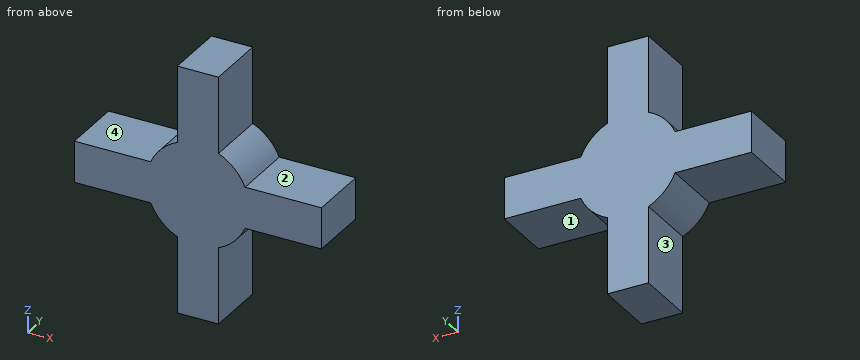
```python
from build123d import *

# Parameters (mm, degrees)
F0_W     = 76.2
F0_H     = 76.2
F2_DEPTH = 19.05
F1_W     = 31.75
F1_H     = 31.75
F3_DEPTH = 19.051
F4_R     = 15.875
F5_DEPTH = 19.05


with BuildPart() as f2:
    # F0 (on Front) → F2 (new body)
    with BuildSketch(Plane.XZ):
        Rectangle(F0_W, F0_H)
    extrude(amount=F2_DEPTH)

    # F1 (on Front) → F3 (cut, through all)
    with BuildSketch(Plane.XZ):
        with Locations((-22.225, 22.225)):
            Rectangle(F1_W, F1_H)
        with Locations((-22.225, -22.225)):
            Rectangle(F1_W, F1_H)
        with Locations((22.225, -22.225)):
            Rectangle(F1_W, F1_H)
        with Locations((22.225, 22.225)):
            Rectangle(F1_W, F1_H)
    extrude(amount=F3_DEPTH, mode=Mode.SUBTRACT)

    # F4 (on Front) → F5 (join)
    with BuildSketch(Plane.XZ):
        Circle(F4_R)
    extrude(amount=F5_DEPTH)


solid = f2.part
```
Geometry: final body of the model. Coordinates: model frame, mm. Face numbers are marked on the shaded views. A direction names the side the tool comes from. Coordinates: 2 decimals unless noted, no trailing zeros. Order: outer loops, then holes, each group sorted by start corner. A loop starts at its lowest first (then second) coordinate and runs counter-clockwise, first axis right, second up.
Item 1: Section query A-A (y = -6.75). Output: boundary loops of the cut face in (x, z) (3 decimals).
Answer:
outline: (-38.1, -6.35) - (-14.55, -6.35) arc R15.875 ccw to (-6.35, -14.55) - (-6.35, -38.1) - (6.35, -38.1) - (6.35, -14.55) arc R15.875 ccw to (14.55, -6.35) - (38.1, -6.35) - (38.1, 6.35) - (14.55, 6.35) arc R15.875 ccw to (6.35, 14.55) - (6.35, 38.1) - (-6.35, 38.1) - (-6.35, 14.55) arc R15.875 ccw to (-14.55, 6.35) - (-38.1, 6.35) - close
Item 2: Section query B-B (z = 28.5). Output: boundary loops of the cut face in (x, y), then the cut area to 3 significant figures.
Answer:
outline: (-6.35, -19.05) - (6.35, -19.05) - (6.35, 0) - (-6.35, 0) - close
area: 242 mm2
Item 3: Contact query for flat-ended pins moving along their axis: P1, Ø1.5, axis at x = 11.5, y = -5.5, coming from the +Z side; P2, Ø9.5, axis at y = -5, z = 22, coming from the -X side; P3, Ø5.5, axis at y = -6.5, z = 29.5, coming from the +X side. Output: stop coordinate, or through.
Answer:
P1: stops at z = 11.68
P2: stops at x = -6.35
P3: stops at x = 6.35
Item 4: Material intervals for line 1 along Z through (x, y) = (15, -3); line 2 along X through (y, z) = (-2, -7.5), sorted ascending.
Answer:
line 1: z = -6.35 to 6.35
line 2: x = -13.99 to 13.99
Item 5: Section query C-C (x = 20). Output: boundary loops of the cut face in (y, z).
Answer:
outline: (-19.05, -6.35) - (0, -6.35) - (0, 6.35) - (-19.05, 6.35) - close
Item 6: Access query for the marked faces 1, 2, 3 and 4. Directions: +Z, -Z, +X, -X, +Y, -Y. A direction counts if a zero-diameter tool reaches every point of the face in a straight line with its end or side. Return the directions, or none.
Answer:
face 1: -Z, +X, +Y, -Y
face 2: +Z, +X, +Y, -Y
face 3: -Z, -X, +Y, -Y
face 4: +Z, -X, +Y, -Y
